```python
from build123d import *

# Parameters (mm, degrees)
EXTRUDE1_DEPTH     = 8.5725
SKETCH2_R          = 1.397
CUT_EXTRUDE1_DEPTH = 6.35


with BuildPart() as part:
    # Sketch1 → Extrude1 (new, symmetric)
    with BuildSketch(Plane(origin=(0, 0, 0), x_dir=(0, 0, -1), z_dir=(1, 0, 0))):
        Polygon((-2.54, 28.575), (-2.54, -2.54), (2.54, -2.54), (2.54, 19.05), (22.225, 19.05), (25.4, 22.225), (25.4, 31.115), (19.05, 31.115), (19.05, 22.225), (6.35, 22.225), (6.35, 31.115), (0, 31.115), align=None)
    extrude(amount=EXTRUDE1_DEPTH, both=True)

    # Sketch2 → Cut-Extrude1 (cut)
    with BuildSketch(Plane(origin=(0, 31.115, 0), x_dir=(-1, 0, 0), z_dir=(0, 1, 0))):
        with Locations(Location((-4.7625, -22.225, 0), (0, 0, 90))):
            Circle(SKETCH2_R)
        with Locations(Location((4.7625, -22.225, 0), (0, 0, 90))):
            Circle(SKETCH2_R)
        with Locations(Location((-4.7625, -3.175, 0), (0, 0, 90))):
            Circle(SKETCH2_R)
        with Locations(Location((4.7625, -3.175, 0), (0, 0, 90))):
            Circle(SKETCH2_R)
    extrude(amount=-CUT_EXTRUDE1_DEPTH, mode=Mode.SUBTRACT)


solid = part.part
```
Could you check a few things on this model? Use its own coordinates, in mm. A direction names the side the tool comes from. Round coordinates to 2 decimals unless told otherwise and drop trailing zeros. Loops run counter-clockwise (first coordinate to the right, second up) from the corner with the lowest first, then second, coordinate; pieces in that order, holes last.
Q1. I want a section at C-C (x = 0.25). Write out the boundary of the cut face in (y, z) (3 decimals).
Q2. I want a section at A-A (y = 24). Write out the boundary of the cut face in (x, z).
Q3. Thinking about a two-plate mould opening in X: for faces 1 (the cylindrical face through (-4.7, 27.98, -23.62)), 2 (the flat face through (0, 31.115, -22)), 3 (the flat face through (-8.572, 22, -8)), which applies, pulls with the +X half, pulls with the -X half, needs draft (parallel to the pull), parting line crosses it, or undercut?
Q4. On a 3-axis mill with a long thin cutter (end or side, diameter ignored), from which of +Z, -Z, +X, -X, +Y, -Y can I reach the whole of each face in a straight line? I mean faces 4 (the flat face through (5, 24.765, -22)), 5 (the flat face through (0, 27, -6.35)), 6 (the flat face through (0, 13, 2.54)), 7 (the flat face through (0, 31.115, -3)), 8 (the flat face through (0, 19.05, -12)). Say none if no direction works.
Q5. For P1, Ø6, axis at x = 6, z = -16, coming from the +Y side (3 decimals); P2, Ø2.5, axis at x = 4.76, z = -22.22, coming from the +Y side (3 decimals); P3, Ø2.5, axis at x = -4.76, z = -22.22, coming from the -Y side, each with a flat end and sliding along its axis, tell me the tip position at first contact or that it passes through.
Q6. Please list where these lines run through material, in increasing order: L1, parallel to Z at x = -5, y = 23; L2, parallel to Z at x = 5.75, y = 11; L3, parallel to Y at x = 6.5, z = -8 (3 decimals).
Q7. I want a section at B-B (y = 29). Give the number of separate pieces and of enclosed holes in the cut face, and give its area (3 significant figures).
Answer below:
1. outline: (-2.54, -2.54) - (19.05, -2.54) - (19.05, -22.225) - (22.225, -25.4) - (31.115, -25.4) - (31.115, -19.05) - (22.225, -19.05) - (22.225, -6.35) - (31.115, -6.35) - (31.115, 0) - (28.575, 2.54) - (-2.54, 2.54) - close
2. outline: (-8.57, -25.4) - (8.57, -25.4) - (8.57, -19.05) - (-8.57, -19.05) - close; (-8.57, -6.35) - (8.57, -6.35) - (8.57, 2.54) - (-8.57, 2.54) - close
3. face 1: undercut
3. face 2: needs draft
3. face 3: pulls with the -X half
4. face 4: +Y
4. face 5: +X, -X, +Y
4. face 6: +Z, +X, -X, +Y, -Y
4. face 7: +Z, -Z, +X, -X, +Y
4. face 8: -Z, +X, -X, -Y
5. P1: stops at y = 22.225
5. P2: stops at y = 24.765
5. P3: stops at y = 19.05
6. L1: z = -25.4 to -19.05, -6.35 to 2.54
6. L2: z = -2.54 to 2.54
6. L3: y = 19.05 to 22.225
7. separate pieces: 2
7. enclosed holes: 4
7. area: 229 mm2
